The model under review builds one solid part; all positions refer to its coordinate system, in mm. Round coordinates to 2 decimals unless told otherwise and drop trailing zeros. Write each loop counter-clockwise with the first axis right and the second up, starting at its lowest first coordinate (ties: lowest second). Pieces come first, ordered by that corner, then holes. Notation, with made-up numbers: (-17.75, 66.5) - (16.25, 66.5) arc R15 cw to (16.25, 95.5) - close; hole circle Ø7 at (-31.5, -27.5). An arc over 180 degrees is marked (long way). Use one line per item in the form item = value.
from build123d import *

# Parameters (mm, degrees)
SM_START                 = -1
SM_BASE_FLANGE_1_DEPTH   = 2
SKETCH_6_R               = 9
SKETCH_6_R_2             = 68.5
CUT_EXTRUDE_1_DEPTH      = 245.769279118
CUT_EXTRUDE_2_DEPTH      = 245.763150821
CUT_EXTRUDE_2_DEPTH_BACK = 245.763150821
CHAMFER_3_SIZE           = 10
CHAMFER_4_SIZE           = 3


# Read off the part's stored shape, not the designer's step: Базовая кромка1
with BuildPart() as part:
    # Базовая кромка1 outline → Базовая кромка1 (new body)
    with BuildSketch(Plane(origin=(0, 0, 0), x_dir=(0, 0, -1), z_dir=(1, 0, 0)).offset(SM_START)):
        with BuildLine():
            ThreePointArc((108, 0), (0, -108), (-108, 0))
            Line((-108, 0), (-108, 150))
            Line((-108, 150), (-148, 150))
            Line((-148, 150), (-148, 146))
            Line((-148, 146), (-168, 146))
            Line((-168, 146), (-168, -10))
            ThreePointArc((-168, -10), (0, -178), (168, -10))
            Line((168, -10), (168, 146))
            Line((168, 146), (148, 146))
            Line((148, 146), (148, 150))
            Line((148, 150), (108, 150))
            Line((108, 150), (108, 0))
        make_face()
    extrude(amount=SM_BASE_FLANGE_1_DEPTH)

    # Эскиз6 → Вырез-Вытянуть1 (cut, through all)
    with BuildSketch(Plane(origin=(1, 0, 0), x_dir=(0, 0, -1), z_dir=(1, 0, 0))):
        with Locations((-135.25, 115)):
            Circle(SKETCH_6_R)
        with Locations((-106.578454425, -83.268214538)):
            Circle(SKETCH_6_R)
        with Locations((0, -135.25)):
            Circle(SKETCH_6_R)
        with Locations((106.578454425, -83.268214538)):
            Circle(SKETCH_6_R)
        with Locations((135.25, 115)):
            Circle(SKETCH_6_R)
        Circle(SKETCH_6_R_2)
        with Locations((-135.25, 25)):
            Circle(SKETCH_6_R)
        with Locations((135.25, 25)):
            Circle(SKETCH_6_R)
    extrude(amount=-CUT_EXTRUDE_1_DEPTH, mode=Mode.SUBTRACT)

    # Эскиз7 → Вырез-Вытянуть2 (cut, two sides: drawn at the far end of the back side and taken through both)
    with BuildSketch(Plane(origin=(0, 0, 0), x_dir=(0, 0, -1), z_dir=(1, 0, 0)).offset(-CUT_EXTRUDE_2_DEPTH_BACK)):
        Polygon((-163, 111), (-168, 106), (-168, 111), (-168, 146), (-163, 146), align=None)
        Polygon((168, 146), (163, 146), (163, 111), (168, 106), (168, 111), align=None)
    extrude(amount=CUT_EXTRUDE_2_DEPTH + CUT_EXTRUDE_2_DEPTH_BACK, mode=Mode.SUBTRACT)

    # Фаска3
    chamfer_3_edges = [part.edges().sort_by_distance(p)[0] for p in [
        (0, 146, 163),
        (0, 146, -163),
    ]]
    chamfer(chamfer_3_edges, length=CHAMFER_3_SIZE)

    # Фаска4
    chamfer_4_edges = [part.edges().sort_by_distance(p)[0] for p in [
        (0, 150, -108),
        (0, 150, 108),
    ]]
    chamfer(chamfer_4_edges, length=CHAMFER_4_SIZE)


solid = part.part
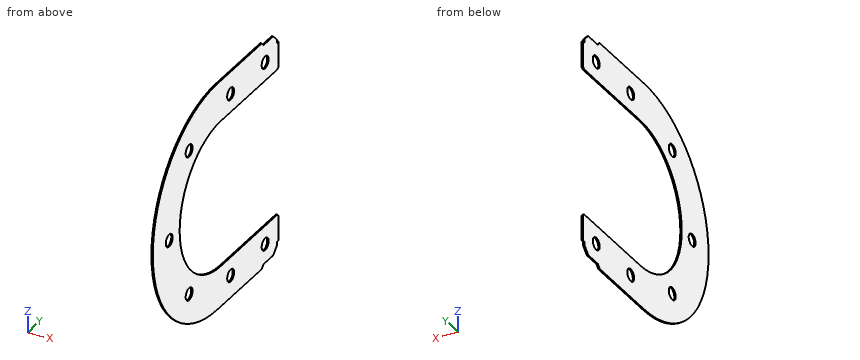
(1) Insertion check: P1, Ø1, axis at x = 0, y = -27.5, coming from the +Z side; P2, Ø1, axis at x = 0, z = -149.5, coming from the +Y side; P3, Ø0.6, axis at x = -0.5, y = 119, coming from the +Z side; P4, Ø23.5, axis at y = -135.25, z = 0, coming from the -X side. Each pin has a flat end and moves straight along its axis. Give the tip position at first contact, or say it passes through.
Geometry results:
P1 = 167.14
P2 = 146
P3 = 163
P4 = -1
(2) Add section D-D on z = -121.5. Write out the cut boundary in (x, y), then the cut area to 3 significant figures.
Geometry results:
outline = (-1, -126.02) - (1, -126.02) - (1, 150) - (-1, 150) - close
area = 552 mm2
(3) Add section C-C on y = -34. Write out the cut boundary in (x, z).
Geometry results:
outline = (-1, -166.28) - (1, -166.28) - (1, -102.51) - (-1, -102.51) - close; (-1, 102.51) - (1, 102.51) - (1, 166.28) - (-1, 166.28) - close
(4) Add section B-B on x = 0. Write out the cut boundary in (y, z), then the cut area to 3 significant figures.
Geometry results:
outline = (-10, -168) - (106, -168) - (111, -163) - (136, -163) - (146, -153) - (146, -148) - (150, -148) - (150, -111) - (147, -108) - (0, -108) arc R108 cw to (0, 108) - (147, 108) - (150, 111) - (150, 148) - (146, 148) - (146, 153) - (136, 163) - (111, 163) - (106, 168) - (-10, 168) arc R168 ccw to start; hole circle Ø18 at (-135.25, 0); hole circle Ø18 at (-83.27, -106.58); hole circle Ø18 at (-83.27, 106.58); hole circle Ø18 at (25, -135.25); hole circle Ø18 at (25, 135.25); hole circle Ø18 at (115, -135.25); hole circle Ø18 at (115, 135.25)
area = 44,900 mm2
(5) To check wall thickness, follow L1, parallel to Z at x = 0.4, y = 135.5; L2, parallel to Y at x = -0.2, z = 135.25; L3, parallel to Z at x = -0.65, y = 91. State the ranges of each line that lie inside material, in increasing order.
Geometry results:
L1 = -163 to -108, 108 to 163
L2 = -109.66 to 16, 34 to 106, 124 to 150
L3 = -168 to -108, 108 to 168
(6) Add section A-A on y = 25. Write out the cut boundary in (x, z).
Geometry results:
outline = (-1, -168) - (1, -168) - (1, -144.25) - (-1, -144.25) - close; (-1, -126.25) - (1, -126.25) - (1, -108) - (-1, -108) - close; (-1, 108) - (1, 108) - (1, 126.25) - (-1, 126.25) - close; (-1, 144.25) - (1, 144.25) - (1, 168) - (-1, 168) - close
